from build123d import *

# Parameters (mm, degrees)
EXTRUDE_1_DEPTH     = 20
SKETCH_2_R          = 1.5
CUT_EXTRUDE_1_DEPTH = 10
SKETCH_4_R          = 1.5
CUT_EXTRUDE_2_DEPTH = 66.76473219
FILLET_1_R          = 2
FILLET_2_R          = 1
FILLET_3_R          = 2


with BuildPart() as part:
    # 草图1 → 凸台-拉伸1 (new body)
    with BuildSketch(Plane.XY):
        Polygon((0, 0), (30, 0), (30, 2), (2, 2), (2, 53), (30, 53), (30, 55), (0, 55), align=None)
    extrude(amount=EXTRUDE_1_DEPTH)

    # 草图2 → 切除-拉伸1 (cut)
    with BuildSketch(Plane.ZY):
        with Locations(Location((10, 41, 0), (0, 0, 270))):
            Circle(SKETCH_2_R)
        with Locations(Location((5.050252532, 45.949747468, 0), (0, 0, 270))):
            Circle(SKETCH_2_R)
        with Locations(Location((14.949747468, 45.949747468, 0), (0, 0, 270))):
            Circle(SKETCH_2_R)
        with Locations(Location((14.949747468, 36.050252532, 0), (0, 0, 270))):
            Circle(SKETCH_2_R)
        with Locations(Location((5.050252532, 36.050252532, 0), (0, 0, 270))):
            Circle(SKETCH_2_R)
    extrude(amount=-CUT_EXTRUDE_1_DEPTH, mode=Mode.SUBTRACT)

    # 草图4 → 切除-拉伸2 (cut, through all)
    with BuildSketch(Plane(origin=(0, 55, 0), x_dir=(1, 0, 0), z_dir=(0, 1, 0))):
        with Locations(Location((18.5, -10, 0), (0, 0, 180))):
            Circle(SKETCH_4_R)
        with Locations(Location((24.5, -10, 0), (0, 0, 180))):
            Circle(SKETCH_4_R)
        with Locations(Location((15.5, -15.196152423, 0), (0, 0, 180))):
            Circle(SKETCH_4_R)
        with Locations(Location((15.5, -4.803847577, 0), (0, 0, 180))):
            Circle(SKETCH_4_R)
    extrude(amount=-CUT_EXTRUDE_2_DEPTH, mode=Mode.SUBTRACT)

    # 圆角1
    fillet_1_edges = [part.edges().sort_by_distance(p)[0] for p in [
        (0, 55, 10),
        (0, 0, 10),
    ]]
    fillet(fillet_1_edges, radius=FILLET_1_R)

    # 圆角2
    fillet_2_edges = [part.edges().sort_by_distance(p)[0] for p in [
        (2, 53, 10),
        (2, 2, 10),
    ]]
    fillet(fillet_2_edges, radius=FILLET_2_R)

    # 圆角3
    fillet_3_edges = [part.edges().sort_by_distance(p)[0] for p in [
        (30, 1, 0),
        (30, 1, 20),
        (30, 54, 20),
        (30, 54, 0),
    ]]
    fillet(fillet_3_edges, radius=FILLET_3_R)


solid = part.part
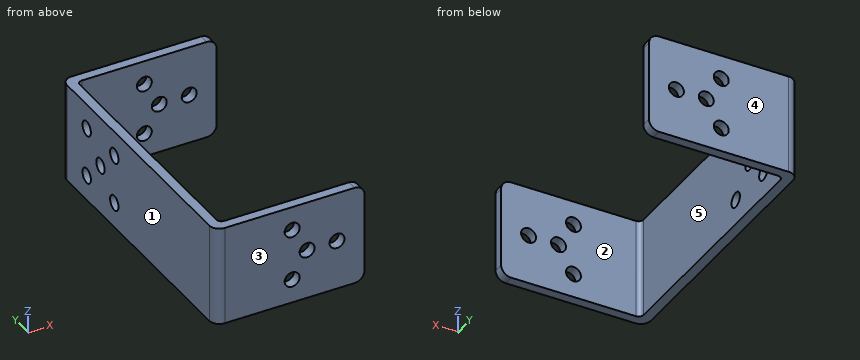
Check sheet for the modelled part. Datum: model origin and axes. Units: mm. Face numbers are marked on the shaded views. A direction names the side the tool comes from. Give positions to 0.01 mm unless a question says otherwise; leave off trailing zeros. Write each loop counter-clockwise with the first axis right and the second up, starting at its lowest first coordinate (ties: lowest second). Pieces come first, ordered by that corner, then holes. Notation, with made-up numbers: (25, -7.75) -> (38, -7.75) arc R18 ccw to (38, 27.25) -> close; hole circle Ø5 at (64.25, 80.5). An arc over 180 degrees is marked (long way). One line per item, written item: value. Start each with the question number.
Item 1: Draft check along Y on the marked faces 1, 2 and 3. Enter one of: +Y half, -Y half, draft (parallel to the pull), parting line (faces both ways), or undercut.
Item 2: Gauge pin test, flat ends, axial feed: pin 1 (5 mm diameter, centred on y = 36.05, z = 5.05, fed in from +X); pin 2 (2.5 mm diameter, centred on x = 18.5, z = 10, fed in from +Y). Record the tip position at first contact, or that the pin passes through.
Item 3: Tool access check on the marked faces 4 and 5. Record the directions out of +Z, -Z, +X, -X, +Y, -Y that give a thin tool (end or side, any length) a straight path to the whole face; none if there is none.
Item 4: Material ranges on probe 1 along Z at (x, y) = (15.5, 54.35); probe 2 along Y at (x, z) = (22, 9); probe 3 along Z at (x, y) = (18.5, 0.6), recorded low to high. Write a range as from..to.
Item 5: Section check B-B on x = 15.5. Record the cut outline in (y, z).
Item 6: Section check A-A on y = 41. Record the cut outline in (x, z), then the cut area to 3 significant figures.
Item 7: Section check C-C on z = 10. State how many separate pieces and enclosed holes the cut face has, then the cut area to 3 significant figures.
Item 8: Section check D-D on x = 10.75. Record the cut outline in (y, z).
Results list:
1. face 1: draft
1. face 2: undercut
1. face 3: -Y half
2. pin 1: x = 2
2. pin 2: through
3. face 4: +Z, -Z, +X, -X, +Y
3. face 5: +Z, -Z, +X
4. probe 1: 0..3.3, 6.3..13.7, 16.7..20
4. probe 2: 0..2, 53..55
4. probe 3: 0..8.5, 11.5..20
5. outline: (0, 0) -> (2, 0) -> (2, 3.3) -> (0, 3.3) -> close; (0, 6.3) -> (2, 6.3) -> (2, 13.7) -> (0, 13.7) -> close; (0, 16.7) -> (2, 16.7) -> (2, 20) -> (0, 20) -> close; (53, 0) -> (55, 0) -> (55, 3.3) -> (53, 3.3) -> close; (53, 6.3) -> (55, 6.3) -> (55, 13.7) -> (53, 13.7) -> close; (53, 16.7) -> (55, 16.7) -> (55, 20) -> (53, 20) -> close
6. outline: (0, 0) -> (2, 0) -> (2, 8.5) -> (0, 8.5) -> close; (0, 11.5) -> (2, 11.5) -> (2, 20) -> (0, 20) -> close
6. area: 34.0 mm²
7. separate pieces: 6
7. enclosed holes: 0
7. area: 191 mm²
8. outline: (0, 0) -> (2, 0) -> (2, 20) -> (0, 20) -> close; (53, 0) -> (55, 0) -> (55, 20) -> (53, 20) -> close
